Here's how the part is built. I have some questions about the finished solid (model axes, mm). A direction names the side the tool comes from. Coordinates: 2 decimals unless noted, no trailing zeros. Loops run counter-clockwise (first coordinate to the right, second up) from the corner with the lowest first, then second, coordinate; pieces in that order, holes last. Notation, with made-up numbers: (-1.75, 75.25) -> (37.25, 75.25) arc R20 cw to (37.25, 105.25) -> close; hole circle Ø8 at (22.25, 66.25). An arc over 180 degrees is marked (long way). Answer as a JSON object with one key per item and string values. Group by question number.
Q1. I want a section at A-A on y = 21.5. Write out the boundary of the cut face in (x, z), then the cut area to 3 significant figures.
Q2. I want a section at C-C on z = -32. Write out the boundary of the cut face in (x, y), then the cut area to 3 significant figures.
Q3. I want a section at B-B on x = -13.95. Write out the boundary of the cut face in (y, z), then the cut area to 3 significant figures.
Q4. Thinking about a two-plate mould opening in Y: for faces 3 (the flat face through (-13.8, -45.2, -122.3)), 4 (the flat face through (-13.8, 44.8, -122.7)), 5 (the flat face through (-13.8, 38.8, 116.7)), which applies, released by +Y, released by -Y, zero draft, split by the parting line, or undercut?
Q5. On a 3-axis mill with a long thin cutter (end or side, diameter ignored), from which of +Z, -Z, +X, -X, +Y, -Y can I reach the whole of each face in a straight line? I mean faces 1 (the flat face through (-13.8, -39.2, 116.3)), 2 (the flat face through (-13.8, 45.2, 122.3)). Say none if no direction works.
Q6. I need wall thicknesses on line 1 (Y direction, x = -14.2, z = -19.5); line 2 (Z direction, x = -13.6, y = 1); line 3 (Y direction, x = -13.6, z = 119.5). Which ranges of each line are inside material? Lowest first, please.
Autodesk Inventor part; units mm, degrees
ref_plane "YZ Plane" through (0, 0, 0) normal (1, 0, 0) x (0, 1, 0)
ref_plane "XZ Plane" through (0, 0, 0) normal (0, 1, 0) x (-1, 0, 0)
ref_plane "XY Plane" through (0, 0, 0) normal (0, 0, 1) x (1, 0, 0)
sketch "Sketch1" plane through (0, 0, 0) normal (1, 0, 0) x (0, 1, 0)
  line L0 (-57.5, 135) -> (57.5, 135)
  line L1 (57.5, 135) -> (57.5, -135)
  line L2 (57.5, -135) -> (-57.5, -135)
  line L3 (-57.5, -135) -> (-57.5, 135)
  line L4 (-57.5, 135) -> (57.5, -135) construction
  line L5 (57.5, 135) -> (-57.5, -135) construction
  circle A0 centre (0, 77.5) radius 3.925
  circle A1 centre (0, -77.5) radius 3.925
  circle A2 centre (-15, 0) radius 5
  line L6 (0, 77.5) -> (0, -77.5) construction
  line L7 (51.5, -129) -> (51.5, 129)
  line L8 (51.5, 129) -> (-51.5, 129)
  line L9 (-51.5, 129) -> (-51.5, -129)
  line L10 (-51.5, -129) -> (51.5, -129)
  point P0 (0, 0)
  dimension "d0" = 155
  dimension "d1" = 7.85
  dimension "d2" = 270
  dimension "d3" = 115
  dimension "d4" = 6
  dimension "d35" = 10
  dimension "d36" = 15
extrude "Extrusion1" add sketch "Sketch1" along normal blind 8 contours L0 L1 L2 L3 | A0 | A1 | L10 L9 L8 L7
extrude "Extrusion2" add sketch "Sketch1" against normal blind 14.4 contours L0 L1 L2 L3
sketch "Sketch2" plane through (8, 0, 0) normal (1, 0, 0) x (0, 0, -1)
  line L0 (135, -57.5) -> (135, 57.5)
  line L1 (135, 57.5) -> (-135, 57.5)
  line L2 (-135, 57.5) -> (-135, -57.5)
  line L3 (-135, -57.5) -> (135, -57.5)
  line L4 (-33.234, -33.234) -> (33.234, -33.234) construction
  line L5 (33.234, -33.234) -> (33.234, 33.234) construction
  line L6 (33.234, 33.234) -> (-33.234, 33.234) construction
  line L7 (-33.234, 33.234) -> (-33.234, -33.234) construction
  line L8 (-33.234, -33.234) -> (33.234, 33.234) construction
  line L9 (33.234, -33.234) -> (-33.234, 33.234) construction
  circle A0 centre (0, 0) radius 47 construction
  circle A1 centre (33.234, 33.234) radius 2.75
  circle A2 centre (-33.234, 33.234) radius 2.75
  circle A3 centre (0, 0) radius 47 construction
  circle A4 centre (-33.234, -33.234) radius 2.75
  circle A5 centre (0, 0) radius 47 construction
  circle A6 centre (33.234, -33.234) radius 2.75
  circle A7 centre (0, 0) radius 47 construction
  point P0 (0, 0)
  point P1 (0, 0)
  dimension "d12" = 94
  dimension "d13" = 5.5
  dimension "d16" = 360
extrude "Extrusion3" cut sketch "Sketch2" against normal through all contours A1 | A2 | A4 | A6
sketch "Sketch3" plane through (0, 0, 0) normal (-1, 0, 0) x (0, 0, 1)
  circle A0 centre (33.234, -33.234) radius 2.75
  circle A1 centre (33.234, 33.234) radius 2.75
  circle A2 centre (-33.234, -33.234) radius 2.75
  circle A3 centre (-33.234, 33.234) radius 2.75
  line L0 (-129, -51.5) -> (129, -51.5)
  line L1 (129, -51.5) -> (129, 51.5)
  line L2 (129, 51.5) -> (-129, 51.5)
  line L3 (-129, 51.5) -> (-129, -51.5)
  circle A4 centre (0, -15) radius 5
  circle A5 centre (-33.234, 33.234) radius 4.5
  circle A6 centre (33.234, 33.234) radius 2.75
  circle A7 centre (33.234, 33.234) radius 4.5
  circle A8 centre (-33.234, -33.234) radius 4.5
  circle A9 centre (33.234, -33.234) radius 4.5
  point P0 (0, 0)
  dimension "d20" = 9
extrude "Extrusion4" cut sketch "Sketch3" against normal blind 3 contours A0 | A1 | A2 | A3 | A5 | A7 | A8 | A9
sketch "Sketch4" plane through (8, 0, 0) normal (1, 0, 0) x (0, 0, -1)
  circle A0 centre (-33.234, -33.234) radius 2.75
  circle A1 centre (-33.234, 33.234) radius 2.75
  circle A2 centre (33.234, -33.234) radius 2.75
  circle A3 centre (33.234, 33.234) radius 2.75
  line L0 (135, -57.5) -> (135, 57.5)
  line L1 (135, 57.5) -> (-135, 57.5)
  line L2 (-135, 57.5) -> (-135, -57.5)
  line L3 (-135, -57.5) -> (135, -57.5)
  circle A4 centre (0, -15) radius 5
  circle A5 centre (0, -15) radius 7.5
  point P0 (0, 0)
  dimension "d24" = 15
extrude "Extrusion5" cut sketch "Sketch4" against normal through all contours A4 | A5
chamfer "Chamfer2" distance 25 angle 45 8 edges at (-7.2, 51.5, -129) (-7.2, -51.5, -129) (-7.2, -51.5, 129) (-7.2, 51.5, 129) (-3.2, 57.5, -135) (-3.2, -57.5, -135) (-3.2, -57.5, 135) (-3.2, 57.5, 135)
sketch "Sketch6" plane through (-14.4, 0, 0) normal (-1, 0, 0) x (0, 0, 1)
  line L0 (110, 57.5) -> (135, 32.5)
  line L1 (110, 57.5) -> (-110, 57.5)
  line L2 (-135, 32.5) -> (-110, 57.5)
  line L3 (-135, 32.5) -> (-135, -32.5)
  line L4 (-110, -57.5) -> (-135, -32.5)
  line L5 (-110, -57.5) -> (110, -57.5)
  line L6 (135, -32.5) -> (110, -57.5)
  line L7 (135, -32.5) -> (135, 32.5)
  line L8 (-129, -26.5) -> (-129, 26.5)
  line L9 (-104, 51.5) -> (-129, 26.5)
  line L10 (-104, 51.5) -> (104, 51.5)
  line L11 (129, 26.5) -> (104, 51.5)
  line L12 (129, 26.5) -> (129, -26.5)
  line L13 (104, -51.5) -> (129, -26.5)
  line L14 (104, -51.5) -> (-104, -51.5)
  line L15 (-129, -26.5) -> (-104, -51.5)
  line L16 (119.5, -42) -> (-119.5, -42)
  line L17 (-119.5, -42) -> (-119.5, 42)
  line L18 (-119.5, 42) -> (119.5, 42)
  line L19 (119.5, 42) -> (119.5, -42)
  circle A0 centre (0, 0) radius 10.3
  line L20 (119.5, -42) -> (-119.5, 42) construction
  line L21 (-119.5, -42) -> (119.5, 42) construction
  circle A1 centre (-119.5, 42) radius 1.5
  circle A2 centre (-119.5, -42) radius 1.5
  circle A3 centre (119.5, -42) radius 1.5
  circle A4 centre (119.5, 42) radius 1.5
  line L22 (-122.5, 45) -> (-116.5, 39)
  dimension "d32" = 3
extrude "Extrusion7" cut sketch "Sketch6" against normal through all contours A2 L16 L17 | L17 L16 A2 | A1 L22 L17 | L17 L22 A1 | L22 L18 A1 | L22 A1 L18 | A3 L19 L16 | L16 L19 A3 | A4 L19 L18 | L18 L19 A4
sketch "Sketch12" plane through (0, 0, 0) normal (-1, 0, 0) x (0, 0, 1)
  circle A0 centre (-77.5, 0) radius 3.925
  circle A1 centre (77.5, 0) radius 3.925
  circle A2 centre (-77.5, 0) radius 11.15
  circle A3 centre (77.5, 0) radius 11.15
  point P0 (0, 0)
  dimension "d61" = 22.3
extrude "Extrusion13" cut sketch "Sketch12" against normal blind 5 contours A0 | A1 | A2 | A3
sketch "Sketch13" plane through (5, 0, -77.5) normal (-1, 0, 0) x (0, 0, 1)
  circle A0 centre (0, 0) radius 11.15
  circle A1 centre (155, 0) radius 11.15
  circle A2 centre (0, 0) radius 8.5
  circle A3 centre (155, 0) radius 8.5
  point P0 (77.5, 0)
  dimension "d64" = 17
  dimension "d65" = 17
extrude "Extrusion14" cut sketch "Sketch13" against normal through all contours A2 | A3
sketch "Sketch14" plane through (0, 0, 0) normal (-1, 0, 0) x (0, 0, 1)
  circle A0 centre (0, -15) radius 7.5
  circle A1 centre (0, -15) radius 9.65
  point P0 (0, 0)
  dimension "d68" = 19.3
extrude "Extrusion15" cut sketch "Sketch14" against normal blind 3
ref_plane "Work Plane1" through (-8.4, 0, 0) normal (-1, 0, 0) x (0, 0, 1)
sketch "Sketch15" plane through (-8.4, 0, 0) normal (-1, 0, 0) x (0, 0, 1)
  circle A0 centre (-119.5, 42) radius 1.5
  line L0 (-120.3667, 45.2345) -> (-117.1322, 44.3678)
  line L1 (-117.1322, 44.3678) -> (-116.2655, 41.1333)
  line L2 (-116.2655, 41.1333) -> (-118.6333, 38.7655)
  line L3 (-118.6333, 38.7655) -> (-121.8678, 39.6322)
  line L4 (-121.8678, 39.6322) -> (-122.7345, 42.8667)
  line L5 (-122.7345, 42.8667) -> (-120.3667, 45.2345)
  line L6 (-135, 32.5) -> (-110, 57.5)
  line L7 (-117.1322, 44.3678) -> (-120.1322, 47.3678)
  line L8 (-121.8678, 39.6322) -> (-124.8678, 42.6322)
  point P0 (0, 0)
  dimension "d72" = 5.8
extrude "Extrusion16" cut sketch "Sketch15" along normal blind 3
mirror "Mirror1" about plane through (0, 0, 0) normal (0, 1, 0) of "Extrusion16"
mirror "Mirror2" about plane through (0, 0, 0) normal (0, 0, 1) of "Extrusion16", "Mirror1"
sketch "Sketch16" plane through (0, 0, 0) normal (-1, 0, 0) x (0, 0, 1)
  circle A0 centre (-21.0923, 23.1558) radius 4
  circle A1 centre (-37.6476, -46.4615) radius 4
  circle A2 centre (0, -15) radius 9.65
  circle A3 centre (77.5, 0) radius 11.15
  circle A4 centre (-77.5, 0) radius 11.15
  line L0 (129, 26.5) -> (104, 51.5)
  line L1 (104, 51.5) -> (-104, 51.5)
  line L2 (-104, 51.5) -> (-129, 26.5)
  line L3 (-129, 26.5) -> (-129, -26.5)
  line L4 (-129, -26.5) -> (-104, -51.5)
  line L5 (-104, -51.5) -> (104, -51.5)
  line L6 (104, -51.5) -> (129, -26.5)
  line L7 (129, -26.5) -> (129, 26.5)
  circle A5 centre (-33.234, -33.234) radius 4.5
  circle A6 centre (33.234, 33.234) radius 4.5
  circle A7 centre (33.234, -33.234) radius 4.5
  circle A8 centre (-33.234, 33.234) radius 4.5
  line L8 (0, 0) -> (0, 21.7983)
  circle A9 centre (21.0923, 23.1558) radius 4
  circle A10 centre (37.6476, -46.4615) radius 4
  dimension "d75" = 8
  dimension "d76" = 8
extrude "Extrusion17" add sketch "Sketch16" along normal up to surface (14.4 mm away) contours A0 | A1 | A9 | A10
sketch "Sketch17" plane through (-14.4, 23.1558, -21.0923) normal (-1, 0, 0) x (0, 0, 1)
  circle A0 centre (0, 0) radius 4
  circle A1 centre (42.1847, 0) radius 4
  circle A2 centre (-16.5553, -69.6173) radius 4
  circle A3 centre (58.7399, -69.6173) radius 4
  circle A4 centre (-16.5553, -69.6173) radius 1.5
  circle A5 centre (58.7399, -69.6173) radius 1.5
  circle A6 centre (0, 0) radius 1.5
  circle A7 centre (42.1847, 0) radius 1.5
  point P0 (21.0923, -23.1558)
  dimension "d79" = 3
extrude "Extrusion18" cut sketch "Sketch17" against normal through all contours A4 | A5 | A6 | A7
chamfer "Chamfer3" distance 3 angle 75 4 edges at (0, -46.4615, -41.6476) (0, 23.1558, -25.0923) (0, 23.1558, 17.0923) (0, -46.4615, 33.6476)
sketch "Sketch18" plane through (-14.4, 0, 0) normal (-1, 0, 0) x (0, 0, 1)
  line L0 (-382.8162, -193.5683) -> (382.8162, -193.5683)
  line L1 (382.8162, -193.5683) -> (382.8162, 193.5683)
  line L2 (382.8162, 193.5683) -> (-382.8162, 193.5683)
  line L3 (-382.8162, 193.5683) -> (-382.8162, -193.5683)
  line L4 (-382.8162, -193.5683) -> (382.8162, 193.5683) construction
  line L5 (382.8162, -193.5683) -> (-382.8162, 193.5683) construction
  circle A0 centre (119.5, -42) radius 1.5
  circle A1 centre (-119.5, -42) radius 1.5
  circle A2 centre (119.5, 42) radius 1.5
  circle A3 centre (-119.5, 42) radius 1.5
  line L6 (110, 57.5) -> (135, 32.5)
  line L7 (110, 57.5) -> (-110, 57.5)
  line L8 (-135, 32.5) -> (-110, 57.5)
  line L9 (-135, 32.5) -> (-135, -32.5)
  line L10 (-110, -57.5) -> (-135, -32.5)
  line L11 (-110, -57.5) -> (110, -57.5)
  line L12 (135, -32.5) -> (110, -57.5)
  line L13 (135, -32.5) -> (135, 32.5)
  line L14 (-129, -26.5) -> (-129, 26.5)
  line L15 (-104, 51.5) -> (-129, 26.5)
  line L16 (-104, 51.5) -> (104, 51.5)
  line L17 (129, 26.5) -> (104, 51.5)
  line L18 (129, 26.5) -> (129, -26.5)
  line L19 (104, -51.5) -> (129, -26.5)
  line L20 (104, -51.5) -> (-104, -51.5)
  line L21 (-129, -26.5) -> (-104, -51.5)
  point P0 (0, 0)
extrude "Extrusion19" cut sketch "Sketch18" against normal blind 22.4 contours L3 L2 L1 L0 | A0 | A1 | A2 | A3 | L6 L13 L12 L11 L10 L9 L8 L7 | L14 L15 L16 L17 L18 L19 L20 L21
extrude "Extrusion20" add sketch "Sketch18" against normal blind 1.2 contours L6 L13 L12 L11 L10 L9 L8 L7
properties part number "CAJA" material "Steel, Mild, Welded"
Result set:
{
 "1": {"outline": "(-14.4, -135) -> (-13.2, -135) -> (-13.2, -129) -> (-14.4, -129) -> close; (-14.4, 129) -> (-13.2, 129) -> (-13.2, 135) -> (-14.4, 135) -> close", "area": "14.4 mm²"},
 "2": {"outline": "(-14.4, -57.5) -> (-13.2, -57.5) -> (-13.2, -51.5) -> (-14.4, -51.5) -> close; (-14.4, 51.5) -> (-13.2, 51.5) -> (-13.2, 57.5) -> (-14.4, 57.5) -> close", "area": "14.4 mm²"},
 "3": {"outline": "(-57.5, -110) -> (-32.5, -135) -> (32.5, -135) -> (57.5, -110) -> (57.5, 110) -> (32.5, 135) -> (-32.5, 135) -> (-57.5, 110) -> close; hole (-51.5, -104) -> (-26.5, -129) -> (26.5, -129) -> (51.5, -104) -> (51.5, 104) -> (26.5, 129) -> (-26.5, 129) -> (-51.5, 104) -> close; hole circle Ø3 at (-42, -119.5); hole circle Ø3 at (-42, 119.5); hole circle Ø3 at (42, -119.5); hole circle Ø3 at (42, 119.5)", "area": "4,450 mm²"},
 "4": {"face 3": "released by -Y", "face 4": "released by +Y", "face 5": "undercut"},
 "5": {"face 1": "+X, -X", "face 2": "+Z, +X, -X, +Y"},
 "6": {"line 1": "y = -57.5 to -51.5, 51.5 to 57.5", "line 2": "z = -135 to -129, 129 to 135", "line 3": "y = -48 to -43.5, -40.5 to -36, 36 to 40.5, 43.5 to 48"}
}
